Work out the finished part from the listing and answer in its coordinate system (mm). A direction names the side the tool comes from. Round coordinates to 2 decimals unless told otherwise and drop trailing zeros. Order: outer loops, then holes, each group sorted by start corner. A loop starts at its lowest first (then second) coordinate and runs counter-clockwise, first axis right, second up.
from build123d import *

# Parameters (mm, degrees)
SKETCH2_W                           = 30.48
SKETCH2_H                           = 152.4
SKETCH4_R                           = 4.89966
BOSS_EXTRUDE1_DEPTH                 = 25.4
BOSS_EXTRUDE1_DEPTH_BACK            = 5.08
F_8_0_199_DIAMETER_HOLE1_AT_2_COUNT = 2
F_8_0_199_DIAMETER_HOLE1_AT_2_PITCH = 50.8
F_8_0_199_DIAMETER_HOLE1_AT_3_COUNT = 2
F_8_0_199_DIAMETER_HOLE1_AT_3_PITCH = 43.994090512
F_8_0_199_DIAMETER_HOLE1_AT_4_COUNT = 2
F_8_0_199_DIAMETER_HOLE1_AT_4_PITCH = 25.4


with BuildPart() as part:
    # Sketch2 → Revolve1 (revolve)
    with BuildSketch(Plane(origin=(0, 0, 0), x_dir=(0, 0, -1), z_dir=(1, 0, 0))):
        with Locations((15.24, 0)):
            Rectangle(SKETCH2_W, SKETCH2_H)
    revolve(axis=Axis((0, -76.2, 0), (0, 1, 0)))


with BuildPart() as body_2:
    # Sketch4 → Boss-Extrude1 (new body, two sides)
    with BuildSketch(Plane(origin=(0, 0, -30.48), x_dir=(-1, 0, 0), z_dir=(0, 0, 1))) as boss_extrude1_sk:
        with BuildLine():
            ThreePointArc((-24.642441225, -6.927272727), (-20.196916389, 0), (-24.642441225, 6.927272727))
            ThreePointArc((-24.642441225, 6.927272727), (-27.423118543, 15.998519166), (-18.090128015, 17.705846349))
            ThreePointArc((-18.090128015, 17.705846349), (-10.809478571, 14.198051615), (-2.729732697, 14.024308028))
            ThreePointArc((-2.729732697, 14.024308028), (0, 14.2875), (2.729732697, 14.024308028))
            ThreePointArc((2.729732697, 14.024308028), (10.809478571, 14.198051615), (18.090128015, 17.705846349))
            ThreePointArc((18.090128015, 17.705846349), (27.423118543, 15.998519166), (24.642441225, 6.927272727))
            ThreePointArc((24.642441225, 6.927272727), (20.196916389, 0), (24.642441225, -6.927272727))
            ThreePointArc((24.642441225, -6.927272727), (27.423118543, -15.998519166), (18.090128015, -17.705846349))
            ThreePointArc((18.090128015, -17.705846349), (10.809478571, -14.198051615), (2.729732697, -14.024308028))
            ThreePointArc((2.729732697, -14.024308028), (0, -14.2875), (-2.729732697, -14.024308028))
            ThreePointArc((-2.729732697, -14.024308028), (-10.809478571, -14.198051615), (-18.090128015, -17.705846349))
            ThreePointArc((-18.090128015, -17.705846349), (-27.423118543, -15.998519166), (-24.642441225, -6.927272727))
        make_face()
        Circle(SKETCH4_R, mode=Mode.SUBTRACT)
    extrude(amount=BOSS_EXTRUDE1_DEPTH)
    extrude(boss_extrude1_sk.sketch, amount=-BOSS_EXTRUDE1_DEPTH_BACK)

    # Sketch10 → 8 _0.199_ Diameter Hole1 (revolve, cut)
    with BuildSketch(Plane(origin=(-21.997045256, 12.7, -35.56), x_dir=(0, 1, 0), z_dir=(1, 0, 0))):
        Polygon((0, 0), (0, 6.598555042), (2.5273, 5.08), (2.5273, 0), align=None)
    f_8_0_199_diameter_hole1 = revolve(axis=Axis((-21.997045256, 12.7, -41.91), (0, 0, 1)), mode=Mode.SUBTRACT)

    # 8 _0.199_ Diameter Hole1 at 2: 8 _0.199_ Diameter Hole1 ×2
    with Locations(*[Vector(0.866025404, -0.5, 0) * (i * F_8_0_199_DIAMETER_HOLE1_AT_2_PITCH) for i in range(1, F_8_0_199_DIAMETER_HOLE1_AT_2_COUNT)]):
        add(f_8_0_199_diameter_hole1, mode=Mode.SUBTRACT)

    # 8 _0.199_ Diameter Hole1 at 3: 8 _0.199_ Diameter Hole1 ×2
    with Locations(*[(i * F_8_0_199_DIAMETER_HOLE1_AT_3_PITCH, 0, 0) for i in range(1, F_8_0_199_DIAMETER_HOLE1_AT_3_COUNT)]):
        add(f_8_0_199_diameter_hole1, mode=Mode.SUBTRACT)

    # 8 _0.199_ Diameter Hole1 at 4: 8 _0.199_ Diameter Hole1 ×2
    with Locations(*[(0, -i * F_8_0_199_DIAMETER_HOLE1_AT_4_PITCH, 0) for i in range(1, F_8_0_199_DIAMETER_HOLE1_AT_4_COUNT)]):
        add(f_8_0_199_diameter_hole1, mode=Mode.SUBTRACT)

    # Combine4: cut part
    add(part.part, mode=Mode.SUBTRACT)


solid = body_2.part
Item 1: Find section B-B (z = -27). Write down the section's boundary in (x, y), plus the area to 3 significant figures.
Item 2: Find section D-D (z = -13). Write down the section's boundary in (x, y), plus the area to 3 significant figures.
Item 3: A tool of negligible diameter and unlimited length cuts with its end or side. For faces 1 (the face through (-24.503, 12.371, -33.056)), 2 (the face through (-12.439, -14.666, -31.194)), from which of +Z, -Z, +X, -X, +Y, -Y can it reach the whole face along a straight path? Write none if from no direction.
Item 4: Find section A-A (x = 0). Write down the section's boundary in (y, z).
Item 5: Given pin 1 (3 mm diameter, centred on x = -22, y = -12.7, fed in from -Z); pin 2 (6.5 mm diameter, centred on x = 22, y = 12.7, fed in from +Z); pin 3 (3 mm diameter, centred on y = -4, z = -21, fed in from +X), each flat-ended and moving along its own axis, determine where each tip first touches the part or whether it passes through.
Item 6: Find section C-C (z = -33.75). State how many separate pieces and enclosed holes the cut face has, plus the area to 3 significant figures.
Item 7: Find the intervals of material crossed by line 1 along X through (y, z) = (12.7, -31.9); line 2 along Y through (x, z) = (0, -31.8); line 3 along X through (y, z) = (-12.5, -15.75), in increasing order.
Model answer:
1. outline: (-24.64, -6.93) arc R6.35 ccw (long way) to (-18.09, -17.71) arc R19.05 cw to (-14.14, -15.33) - (-14.14, 15.33) arc R19.05 cw to (-18.09, 17.71) arc R6.35 ccw (long way) to (-24.64, 6.93) arc R7.62 cw to start; (14.14, -15.33) arc R19.05 cw to (18.09, -17.71) arc R6.35 ccw (long way) to (24.64, -6.93) arc R7.62 cw to (24.64, 6.93) arc R6.35 ccw (long way) to (18.09, 17.71) arc R19.05 cw to (14.14, 15.33) - close
1. area: 784 mm2
2. outline: (-27.57, -15.75) - (-27.57, -9.65) arc R6.35 ccw to start; (-27.57, 9.65) - (-27.57, 15.75) arc R6.35 ccw to start; (27.57, -15.75) arc R6.35 ccw to (27.57, -9.65) - close; (27.57, 9.65) arc R6.35 ccw to (27.57, 15.75) - close
2. area: 12.8 mm2
3. face 1: -Z
3. face 2: +Z, -Z, -Y
4. outline: (-14.29, -35.56) - (-4.9, -35.56) - (-4.9, -30.48) - (-14.29, -30.48) - close; (4.9, -35.56) - (14.29, -35.56) - (14.29, -30.48) - (4.9, -30.48) - close
5. pin 1: stops at z = -29.86
5. pin 2: stops at z = -17.07
5. pin 3: stops at x = 22.54
6. separate pieces: 1
6. enclosed holes: 5
6. area: 1,430 mm2
7. line 1: x = -28.35 to -24.52, -19.47 to 19.47, 24.52 to 28.35
7. line 2: y = -14.29 to -4.9, 4.9 to 14.29
7. line 3: x = -28.34 to -26.1, 26.1 to 28.34
